```python
from build123d import *

# Parameters (mm, degrees)
SKETCH1_W          = 88.9
SKETCH1_H          = 88.9
BASE_EXTRUDE_DEPTH = 19.05
CUT_EXTRUDE1_DEPTH = 89.9
CUT_EXTRUDE2_DEPTH = 89.9


with BuildPart() as part:
    # Sketch1 → Base-Extrude (new body)
    with BuildSketch(Plane(origin=(0, 0, 0), x_dir=(1, 0, 0), z_dir=(0, 1, 0))):
        Rectangle(SKETCH1_W, SKETCH1_H)
    extrude(amount=BASE_EXTRUDE_DEPTH)

    # Sketch2 → Cut-Extrude1 (cut, through all)
    with BuildSketch(Plane.XY.offset(44.45)):
        Polygon((6.35, 9.525), (-6.35, 9.525), (-3.975150773, 19.05), (3.975150773, 19.05), align=None)
    extrude(amount=-CUT_EXTRUDE1_DEPTH, mode=Mode.SUBTRACT)

    # Sketch3 → Cut-Extrude2 (cut, through all)
    with BuildSketch(Plane(origin=(44.45, -3.538159269, -0.664564519), x_dir=(0, 0, -1), z_dir=(1, 0, 0))):
        Polygon((5.685435481, 13.063159269), (-7.014564519, 13.063159269), (-4.639715292, 22.588159269), (3.310586254, 22.588159269), align=None)
    extrude(amount=-CUT_EXTRUDE2_DEPTH, mode=Mode.SUBTRACT)


solid = part.part
```
Geometry: final body of the model. Coordinates: model frame, mm. A direction names the side the tool comes from. Give positions to 0.01 mm unless a question says otherwise; leave off trailing zeros. Order: outer loops, then holes, each group sorted by start corner. A loop starts at its lowest first (then second) coordinate and runs counter-clockwise, first axis right, second up. Notation, with made-up numbers: (64.25, 24) -> (69.25, 24) arc R21 cw to (69.25, 46) -> close; hole circle Ø5 at (-10, 50). An arc over 180 degrees is marked (long way). Write each question's results on one line, items separated by ' | '. Start each with the question number.
1) Section A-A (y = 17.5). Return loops of the section in (x, z), then the cut area to 3 significant figures.
2) Set-up query: faces 1 (the flat face through (5.146, 14.354, -23.929)), 2 (the flat face through (24.5, 14.22, 5.18)), 3 (the flat face through (-1, 9, -44.45)). Return all of +Z, -Z, +X, -X, +Y, -Y with unobstructed straight access to the full face (end or side cutting, diameter ignored); none if empty.
3) Line query: line 1 (Z direction, x = 19, y = 12); line 2 (Z direction, x = 5.5, y = 16.75). Output: solid intervals per line, ascending. Write a range as from..to.
4) Section C-C (z = -22.5). Return loops of the section in (x, y) (3 decimals).
5) Section B-B (x = 39). Return loops of the section in (y, z) (3 decimals), then the cut area to 3 significant figures.
6) Section D-D (y = 11.25). Return loops of the section in (x, z).
7) Draft query along X for faces 4 (the flat face through (-44.45, 9, 1)), 5 (the flat face through (44.45, 9, 1)), 6 (the flat face through (24, 19.05, -24)), 7 (the flat face through (5.146, 14.354, 24.496)). Return one class per face: pulls with the +X half, pulls with the -X half, needs draft (parallel to the pull), parting line crosses it, or undercut.
Calculated:
1) outline: (-44.45, -44.45) -> (-4.36, -44.45) -> (-4.36, -4.36) -> (-44.45, -4.36) -> close; (-44.45, 4.36) -> (-4.36, 4.36) -> (-4.36, 44.45) -> (-44.45, 44.45) -> close; (4.36, -44.45) -> (44.45, -44.45) -> (44.45, -4.36) -> (4.36, -4.36) -> close; (4.36, 4.36) -> (44.45, 4.36) -> (44.45, 44.45) -> (4.36, 44.45) -> close | area: 6,430 mm2
2) face 1: +Z, -Z | face 2: +X, -X | face 3: -Z, +X, -X, +Y, -Y
3) line 1: -44.45..-5.73, 5.73..44.45 | line 2: -44.45..-4.55, 4.55..44.45
4) outline: (-44.45, 0) -> (44.45, 0) -> (44.45, 19.05) -> (3.975, 19.05) -> (6.35, 9.525) -> (-6.35, 9.525) -> (-3.975, 19.05) -> (-44.45, 19.05) -> close
5) outline: (0, -44.45) -> (19.05, -44.45) -> (19.05, -3.975) -> (9.525, -6.35) -> (9.525, 6.35) -> (19.05, 3.975) -> (19.05, 44.45) -> (0, 44.45) -> close | area: 1,600 mm2
6) outline: (-44.45, -44.45) -> (-5.92, -44.45) -> (-5.92, -5.92) -> (-44.45, -5.92) -> close; (-44.45, 5.92) -> (-5.92, 5.92) -> (-5.92, 44.45) -> (-44.45, 44.45) -> close; (5.92, -44.45) -> (44.45, -44.45) -> (44.45, -5.92) -> (5.92, -5.92) -> close; (5.92, 5.92) -> (44.45, 5.92) -> (44.45, 44.45) -> (5.92, 44.45) -> close
7) face 4: pulls with the -X half | face 5: pulls with the +X half | face 6: needs draft | face 7: undercut
